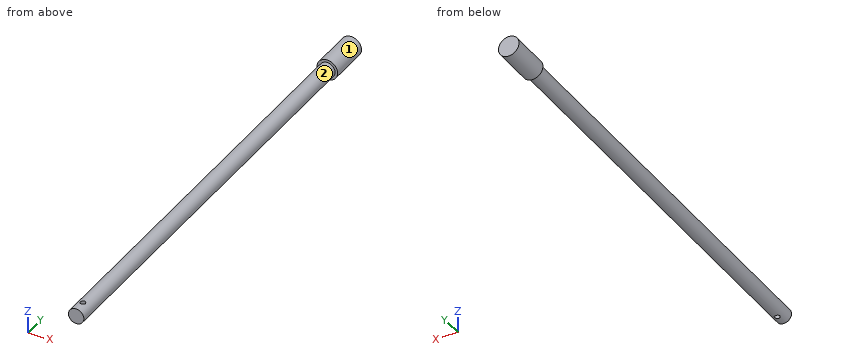
```python
from build123d import *

# Parameters (mm, degrees)
F0_R     = 3.175
F0_R_2   = 2.38125
F1_DEPTH = 12.7
F2_DEPTH = 146.05
F3_R     = 0.79375
F4_DEPTH = 3.175


with BuildPart() as f1:
    # F0 (on Front) → F1 (new body)
    with BuildSketch(Plane.XZ):
        Circle(F0_R)
        Circle(F0_R_2, mode=Mode.SUBTRACT)
    extrude(amount=F1_DEPTH)

    # F0 (on Front) → F2 (join)
    with BuildSketch(Plane.XZ):
        Circle(F0_R_2)
    extrude(amount=F2_DEPTH)

    # F3 (on Top) → F4 (cut, symmetric)
    with BuildSketch(Plane.XY):
        with Locations((0, -142.5194)):
            Circle(F3_R)
    extrude(amount=F4_DEPTH, both=True, mode=Mode.SUBTRACT)


solid = f1.part
```
CAD build for the part. Positions are in the model's coordinates, mm. Face numbers are marked on the shaded views. A direction names the side the tool comes from. Round coordinates to 2 decimals unless told otherwise and drop trailing zeros. Write each loop counter-clockwise with the first axis right and the second up, starting at its lowest first coordinate (ties: lowest second). Pieces come first, ordered by that corner, then holes. Notation, with made-up numbers: (83.5, 25) - (88.5, 25) arc R25 ccw to (88.5, 44) - close; hole circle Ø10 at (-34.5, -16). An arc over 180 degrees is marked (long way). Return JSON: item names as keys, results as strings. Group by question number.
Item 1: Flat gauge pins, fed straight in: pin 1 Ø1.5 at (y, z) = (-41.5, 0) entering from +X; pin 2 Ø1.8 at (x, y) = (0, -142.52) entering from +Z; pin 3 Ø1 at (y, z) = (-26, -0.5) entering from -X; pin 4 Ø3 at (x, z) = (-2.5, -2) entering from +Y. Where does each tip first touch, or does it go through?
Item 2: Band-saw the part on B-B on y = -48.5. List the corners of the cut face in (x, z).
Item 3: 3-axis set-ups, long thin cutter, end or side, ignore diameter. For the marked faces 1 and 2: which of +Z, -Z, +X, -X, +Y, -Y reach the whole face in a straight line?
Item 4: Probe probe 1 along Y at (x, z) = (0, 0.9); probe 2 along Y at (x, z) = (-0.5, 2.5); probe 3 along X at (y, z) = (-77, 0.25). List the from-to ranges inside material, lowest first.
Resolved:
{
 "1": {"pin 1": "stops at x = 2.38", "pin 2": "stops at z = 2.38", "pin 3": "stops at x = -2.38", "pin 4": "stops at y = 0"},
 "2": {"outline": "circle Ø4.76 at (0, 0)"},
 "3": {"face 1": "+Y, -Y", "face 2": "-Y"},
 "4": {"probe 1": "y = -146.05 to -143.31, -141.73 to 0", "probe 2": "y = -12.7 to 0", "probe 3": "x = -2.37 to 2.37"}
}
